from build123d import *

# Parameters (mm, degrees)
F0_W     = 127
F0_H     = 127
F1_DEPTH = 127
F2_SIZE  = 5.08
F4_DEPTH = 127


with BuildPart() as f1:
    # F0 (on Front) → F1 (new body)
    with BuildSketch(Plane.XZ):
        with Locations((-0.227161, 13.688557)):
            Rectangle(F0_W, F0_H)
    extrude(amount=F1_DEPTH)

    # F2
    f2_edges = [f1.edges().sort_by_distance(p)[0] for p in [
        (-0.227161, -127, 77.188557),
        (63.272839, -63.5, 77.188557),
        (63.272839, -63.5, -49.811443),
        (-0.227161, -127, -49.811443),
        (-63.727161, -63.5, -49.811443),
        (-0.227161, 0, -49.811443),
        (-63.727161, -63.5, 77.188557),
        (-0.227161, 0, 77.188557),
        (-63.727161, 0, 13.688557),
        (63.272839, 0, 13.688557),
        (-63.727161, -127, 13.688557),
        (63.272839, -127, 13.688557),
    ]]
    chamfer(f2_edges, length=F2_SIZE)

    # F3 (on face) → F4 (cut)
    with BuildSketch(Plane.XZ.offset(127)):
        with BuildLine():
            Line((17.552839, 11.196052), (17.552839, 36.596052))
            ThreePointArc((17.552839, 36.596052), (-25.807673, 54.556565), (-7.847161, 11.196052))
            Line((-7.847161, 11.196052), (17.552839, 11.196052))
        make_face()
    extrude(amount=-F4_DEPTH, mode=Mode.SUBTRACT)


solid = f1.part
Read the model definition and answer for the solid it produces. Units are mm, in the model's axes. Coordinates: 2 decimals unless noted, no trailing zeros. Order: outer loops, then holes, each group sorted by start corner. A loop starts at its lowest first (then second) coordinate and runs counter-clockwise, first axis right, second up. Notation, with made-up numbers: (12.25, 19) -> (50.25, 19) arc R21 cw to (50.25, 49) -> close; hole circle Ø9 at (-17.75, -36.5). An arc over 180 degrees is marked (long way). Answer as a JSON object with one key per item and string values.
1) A cutting plane is placed at B-B, the plane x = -19.5. Determine the outline of the cut face in (y, z).
Model answer:
{"outline": "(-127, -44.73) -> (-121.92, -49.81) -> (-5.08, -49.81) -> (0, -44.73) -> (0, 14.03) -> (-127, 14.03) -> close; (-127, 59.17) -> (0, 59.17) -> (0, 72.11) -> (-5.08, 77.19) -> (-121.92, 77.19) -> (-127, 72.11) -> close"}
2) A cutting plane is placed at C-C, the plane z = 26. Determine the outline of the cut face in (x, y).
Model answer:
{"outline": "(-63.73, -121.92) -> (-58.65, -127) -> (-30.93, -127) -> (-30.93, 0) -> (-58.65, 0) -> (-63.73, -5.08) -> close; (17.55, -127) -> (58.19, -127) -> (63.27, -121.92) -> (63.27, -5.08) -> (58.19, 0) -> (17.55, 0) -> close"}
3) Consider line 1 along Z through (x, y) = (-8, -25.5); line 2 along X through (y, z) = (-48, 37); line 3 along Z through (x, y) = (7, -26). Determine where each line is inside the solid, lowest interval first. Write a range as from..to.
Model answer:
{"line 1": "z = -49.81..11.2, 62..77.19", "line 2": "x = -63.73..-33.24, 17.55..63.27", "line 3": "z = -49.81..11.2, 57.2..77.19"}
4) This flat-tipped pin is pushed along its axis until it touches: pin 1 (4 mm diameter, centred on x = 1, z = 57.5, fed in from +Y). Where does it stop, or does it pass through?
Model answer:
{"pin 1": "passes through"}
5) A cutting plane is placed at A-A, the plane y = -32. Determine the outline of the cut face in (x, z).
Model answer:
{"outline": "(-63.73, -44.73) -> (-58.65, -49.81) -> (58.19, -49.81) -> (63.27, -44.73) -> (63.27, 72.11) -> (58.19, 77.19) -> (-58.65, 77.19) -> (-63.73, 72.11) -> close; hole (-7.85, 11.2) -> (17.55, 11.2) -> (17.55, 36.6) arc R25.4 ccw (long way) to start"}
6) The mould has two halves that part along X. Classify faces 1 (the face through (5, -64, 11.196)), 2 (the face through (59.727, -3.14, -46.337)), 3 (the face through (-1, -63, -49.811)), 4 (the face through (-60.18, -3.14, -46.34)): released by +X, released by -X, zero draft, split by the parting line, or undercut.
Model answer:
{"face 1": "undercut", "face 2": "released by +X", "face 3": "zero draft", "face 4": "released by -X"}
